For this review, use the dimensioned drawing (mm, ordinates from the lowest corner) and the shaded views. A direction names the side the tool comes from. Coordinates: 2 decimals unless noted, no trailing zeros. Loops run counter-clockwise (first coordinate to the right, second up) from the corner with the lowest first, then second, coordinate; pieces in that order, holes last.
1. Mouldability with a two-part tool opening along X and no side actions: class the marked faces 1, 2 and 3 as pulls with the +X half, pulls with the -X half, needs draft (parallel to the pull), parting line crosses it, or undercut.
2. Clearance check with flat-ended pins moving along their axes: P1, Ø1.5, axis at x = 8.5, z = 12.5, coming from the -Y side; P2, Ø5, axis at y = 4.5, z = 10.5, coming from the -X side; P3, Ø4, axis at x = 4, y = 11.5, coming from the +Z side; P4, Ø5, axis at y = 12.5, z = 2, coming from the -X side. State where each tip first meets the part, or that it passes through.
3. Machinability: for the marked faces 4, 5, 6 and 7, which of the approach directions +Z, -Z, +X, -X, +Y, -Y give a long, thin tool a straight path to every point of the face, cutting with its end or side? Answer none if there is none.
4. Take a section at D-D, the plane x = 2.25. State the section outline as (y, z) points.
5. Take a section at A-A, the plane x = 7.4. State the section outline as (y, z) points (3 decimals).
6. To check wall thickness, follow probe 1 along Y at (x, z) = (7.4, 5.5) (3 decimals); probe 2 along X at (y, z) = (7.5, 5); probe 3 along Z at (x, y) = (5.5, 14). State the ranges of each line that lie inside material, in increasing order.
7. Take a section at C-C, the plane z = 2. State the section outline as (x, y) points (3 decimals), then the cut area to 3 significant figures.
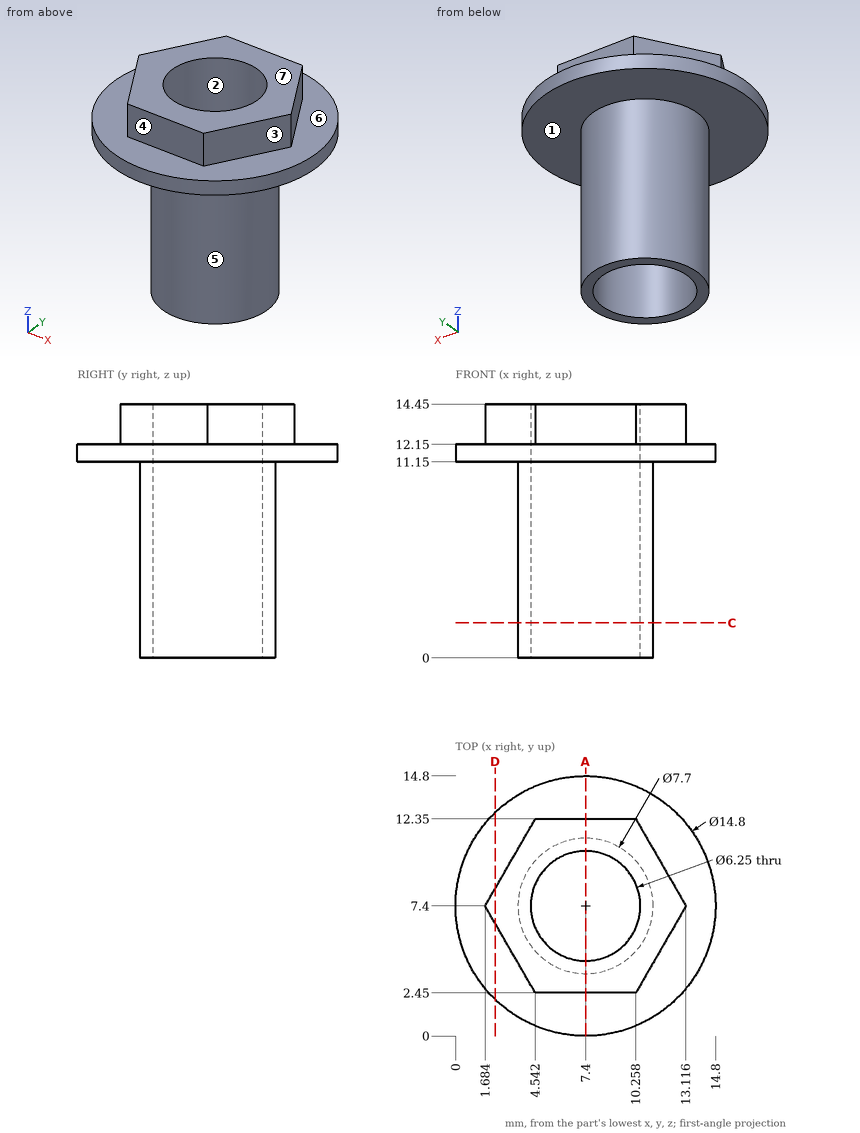
Results list:
1. face 1: needs draft
1. face 2: undercut
1. face 3: pulls with the +X half
2. P1: stops at y = 0.01
2. P2: stops at x = 0.02
2. P3: stops at z = 14.45
2. P4: stops at x = 4.56
3. face 4: +Z, +X, -X, -Y
3. face 5: -Z
3. face 6: +Z
3. face 7: +Z, +X, -X, +Y, -Y
4. outline: (2.09, 11.15) - (12.71, 11.15) - (12.71, 12.15) - (8.38, 12.15) - (8.38, 14.45) - (6.42, 14.45) - (6.42, 12.15) - (2.09, 12.15) - close
5. outline: (0, 11.15) - (3.55, 11.15) - (3.55, 0) - (4.275, 0) - (4.275, 14.45) - (2.45, 14.45) - (2.45, 12.15) - (0, 12.15) - close; (10.525, 0) - (11.25, 0) - (11.25, 11.15) - (14.8, 11.15) - (14.8, 12.15) - (12.35, 12.15) - (12.35, 14.45) - (10.525, 14.45) - close
6. probe 1: y = 3.55 to 4.275, 10.525 to 11.25
6. probe 2: x = 3.55 to 4.28, 10.52 to 11.25
6. probe 3: z = 11.15 to 12.15
7. outline: circle Ø7.7 at (7.4, 7.4); hole circle Ø6.25 at (7.4, 7.4)
7. area: 15.9 mm2
